Input: dimensioned drawing with shaded views. Units: mm. Origin: part minimum x, y, z. A direction names the side the tool comes from. Give positions to 0.01 mm unless a question says otherwise; leave off trailing zeros. Loops run counter-clockwise (first coordinate to the right, second up) from the corner with the lowest first, then second, coordinate; pieces in that order, holes last. Notation, with made-up numbers: (58, 53) -> (108, 53) arc R20 cw to (108, 69) -> close; hole circle Ø4 at (64, 36). An arc over 180 degrees is marked (long way). Answer in a Markdown table with one row per item. Add a question column.
1) First-contact query: P1, Ø1, axis at x = 16.5, z = 27, coming from the -Y side. Flat tip, straight axial feed; report the tip coordinate or a pass-through.
2) Section query C-C (z = 17). Return the cut outline in (x, y), plus the area to 3 significant figures.
3) Line query: line 1 (X direction, y = 24.6, z = 20.25); line 2 (Z direction, x = 11, y = 13.5); line 3 (Y direction, x = 3, z = 1.15). Output: solid intervals per line, ascending. Write a range as from..to.
4) Draft query along Z for the marked faces 3, 4, 5 and 6. Return one class per face: +Z half, -Z half, draft (parallel to the pull), parting line (faces both ways), or undercut.
5) Section query D-D (y = 21.75). Return the cut outline in (x, z), plus the area to 3 significant figures.
6) Access query for the marked faces 1 and 2. Directions: +Z, -Z, +X, -X, +Y, -Y. A direction counts if a zero-diameter tool reaches every point of the face in a straight line with its end or side. Return the directions, or none.
7) Section query A-A (y = 10). Return the cut outline in (x, z).
8) Section query B-B (x = 17). Return the cut outline in (y, z), plus the area to 3 significant figures.
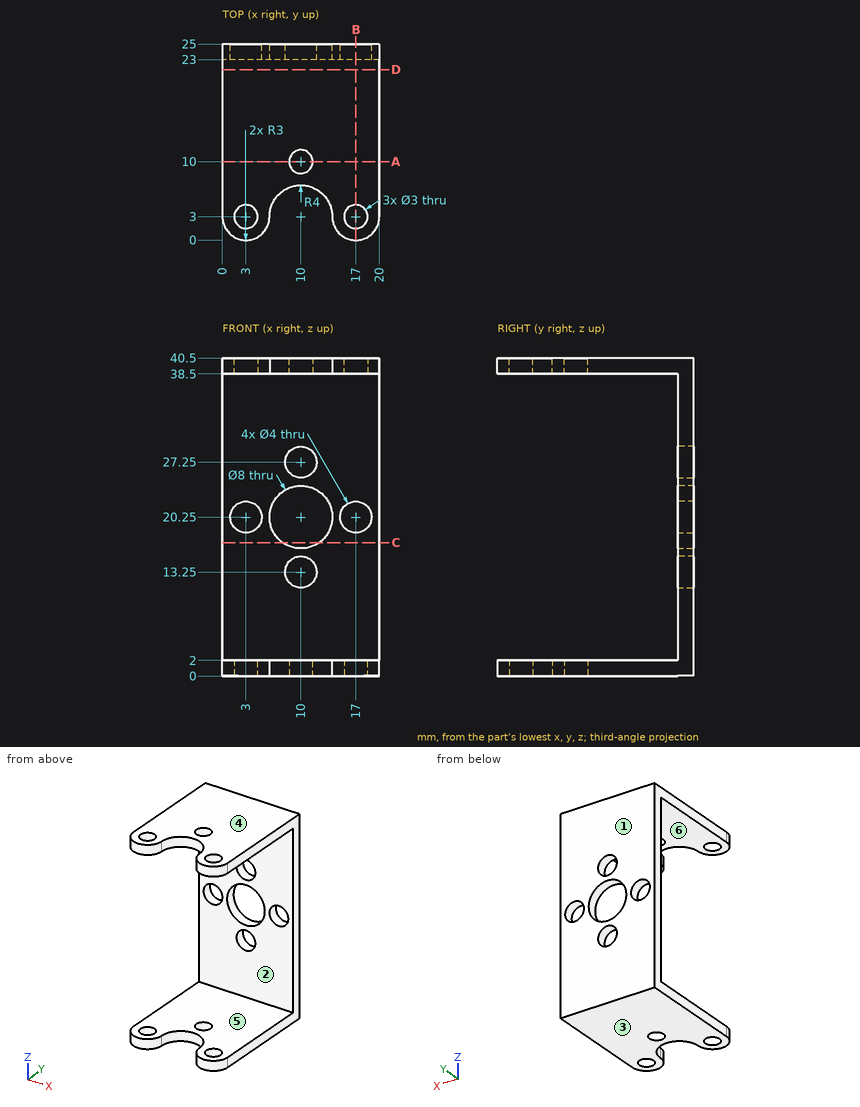
Evaluation:
| question | item | result |
|---|---|---|
| 1 | P1 | y = 23 |
| 2 | outline | (0, 23) -> (7.67, 23) -> (7.67, 25) -> (0, 25) -> close; (12.33, 23) -> (20, 23) -> (20, 25) -> (12.33, 25) -> close |
| 2 | area | 30.7 mm² |
| 3 | line 1 | 0..1, 5..6, 14..15, 19..20 |
| 3 | line 2 | 0..2, 38.5..40.5 |
| 3 | line 3 | 0..1.5, 4.5..25 |
| 4 | face 3 | -Z half |
| 4 | face 4 | +Z half |
| 4 | face 5 | undercut |
| 4 | face 6 | undercut |
| 5 | outline | (0, 0) -> (20, 0) -> (20, 2) -> (0, 2) -> close; (0, 38.5) -> (20, 38.5) -> (20, 40.5) -> (0, 40.5) -> close |
| 5 | area | 80.0 mm² |
| 6 | face 1 | +Z, -Z, +X, -X, +Y |
| 6 | face 2 | +X, -X, -Y |
| 7 | outline | (0, 0) -> (8.5, 0) -> (8.5, 2) -> (0, 2) -> close; (0, 38.5) -> (8.5, 38.5) -> (8.5, 40.5) -> (0, 40.5) -> close; (11.5, 0) -> (20, 0) -> (20, 2) -> (11.5, 2) -> close; (11.5, 38.5) -> (20, 38.5) -> (20, 40.5) -> (11.5, 40.5) -> close |
| 8 | outline | (0, 0) -> (1.5, 0) -> (1.5, 2) -> (0, 2) -> close; (0, 38.5) -> (1.5, 38.5) -> (1.5, 40.5) -> (0, 40.5) -> close; (4.5, 0) -> (25, 0) -> (25, 18.25) -> (23, 18.25) -> (23, 2) -> (4.5, 2) -> close; (4.5, 38.5) -> (23, 38.5) -> (23, 22.25) -> (25, 22.25) -> (25, 40.5) -> (4.5, 40.5) -> close |
| 8 | area | 153 mm² |
